```python
from build123d import *

# Parameters (mm, degrees)
EXTRUDE_1_DEPTH       = 27
EXTRUDE_2_DEPTH       = 7
CUT_EXTRUDE_START     = -19
CUT_EXTRUDE_3_DEPTH   = 38
SKETCH_2_R            = 6
CUT_EXTRUDE_3_2_DEPTH = 61.934390946


# Read off the part's stored shape, not the designer's step: 切除-拉伸-薄壁3
with BuildPart() as part:
    # 草图1 → 凸台-拉伸1 (new, symmetric)
    with BuildSketch(Plane.XY):
        Polygon((23, 12), (0, 0), (-23, 12), (-50, 12), (-50, 0), (-32, 0), (-32, -10), (32, -10), (32, 0), (50, 0), (50, 12), align=None)
        Polygon((-32, 0), (-50, 0), (-42, -10), (-32, -10), align=None)
        Polygon((42, -10), (50, 0), (32, 0), (32, -10), align=None)
    extrude(amount=EXTRUDE_1_DEPTH, both=True)

    # 草图1<4> → 凸台-拉伸2 (add, symmetric)
    with BuildSketch(Plane.XY):
        Polygon((0, 12), (0, 0), (23, 12), align=None)
        Polygon((-23, 12), (0, 0), (0, 12), align=None)
    extrude(amount=EXTRUDE_2_DEPTH, both=True)

    # Cut-Extrude 3 outline → Cut-Extrude 3 (cut)
    with BuildSketch(Plane.XY.offset(CUT_EXTRUDE_START)):
        Polygon((-32, 0), (-50, 0), (-42, -10), (-32, -10), align=None)
    cut_extrude_3 = extrude(amount=CUT_EXTRUDE_3_DEPTH, mode=Mode.SUBTRACT)

    # 镜向1: Cut-Extrude 3 across plane
    add(cut_extrude_3.mirror(Plane(origin=(0, 0, 0), x_dir=(0, 0, 1), z_dir=(1, 0, 0))), mode=Mode.SUBTRACT)

    # 草图2 → Cut-Extrude 3 2 (cut, through all)
    with BuildSketch(Plane(origin=(0, 12, 0), x_dir=(1, 0, 0), z_dir=(0, 1, 0))):
        with Locations(Location((42, 0, 0), (0, 0, 180))):
            Circle(SKETCH_2_R)
        with Locations(Location((-42, 0, 0), (0, 0, 90))):
            Circle(SKETCH_2_R)
    extrude(amount=-CUT_EXTRUDE_3_2_DEPTH, mode=Mode.SUBTRACT)


solid = part.part
```
Part model, mm, in its own coordinate system. A direction names the side the tool comes from. Round coordinates to 2 decimals unless told otherwise and drop trailing zeros. Loops run counter-clockwise (first coordinate to the right, second up) from the corner with the lowest first, then second, coordinate; pieces in that order, holes last.
1. Drill centre lines: line 1 along X through (y, z) = (9, 1.5); line 2 along Z through (x, y) = (-42, 9.75); line 3 along X through (y, z) = (11.25, 16.5). Where is each one in solid material? Low to high.
Solutions:
line 1: x = -50 to -47.81, -36.19 to 36.19, 47.81 to 50
line 2: z = -27 to -6, 6 to 27
line 3: x = -50 to -21.56, 21.56 to 50
2. Slice it at B-B (y = -8). Give the cut face in (x, z), and give its area (3 significant figures).
Solutions:
outline: (-43.6, -27) - (43.6, -27) - (43.6, -19) - (32, -19) - (32, 19) - (43.6, 19) - (43.6, 27) - (-43.6, 27) - (-43.6, 19) - (-32, 19) - (-32, -19) - (-43.6, -19) - close
area: 3,830 mm2
3. Flat gauge pins, fed straight in: pin 1 (1 mm diameter, centred on y = -1, z = 3, fed in from -X); pin 2 (19 mm diameter, centred on x = 42, z = 0, fed in from -Y); pin 3 (3.5 mm diameter, centred on x = -11, y = 8, fed in from -Z). Where does each tip first touch, or does it go through?
Solutions:
pin 1: stops at x = -32
pin 2: stops at y = 0
pin 3: stops at z = -7
4. Slice it at A-A (z = 0). Give the cut face in (x, y).
Solutions:
outline: (-50, 0) - (-48, 0) - (-48, 12) - (-50, 12) - close; (-36, 0) - (-32, 0) - (-32, -10) - (32, -10) - (32, 0) - (36, 0) - (36, 12) - (-36, 12) - close; (48, 0) - (50, 0) - (50, 12) - (48, 12) - close
5. Two-plate mould, pull along Z, no slides. Class faces 4 (the face through (-1, -1, -27)), 5 (the face through (0, 7, 7)), 6 (the face through (-46, -5, -23)), 7 (the face through (-37, 0, -4)): pulls with the +Z half, pulls with the -Z half, needs draft (parallel to the pull), parting line crosses it, or undercut.
Solutions:
face 4: pulls with the -Z half
face 5: pulls with the +Z half
face 6: needs draft
face 7: undercut
6. Slice it at C-C (x = -10). Give the cut face in (y, z), and give its area (3 significant figures).
Solutions:
outline: (-10, -27) - (5.22, -27) - (5.22, -7) - (12, -7) - (12, 7) - (5.22, 7) - (5.22, 27) - (-10, 27) - close
area: 917 mm2
7. 3-axis set-ups, long thin cutter, end or side, ignore diameter. For faces 1 (the face through (-32, -5, 0)), 2 (the face through (32, -5, 0)), 3 (the face through (0, 7, -7)): which of +Z, -Z, +X, -X, +Y, -Y reach the whole face in a straight line?
Solutions:
face 1: -X, -Y
face 2: +X, -Y
face 3: -Z, +Y
8. Slice it at D-D (z = -9). Give the cut face in (x, y), and give its area (3 significant figures).
Solutions:
outline: (-50, 0) - (-32, 0) - (-32, -10) - (32, -10) - (32, 0) - (50, 0) - (50, 12) - (23, 12) - (0, 0) - (-23, 12) - (-50, 12) - close
area: 1,560 mm2
